Can you work these out from the drawing? Everything is in mm from the part's minimum corner. A direction names the side the tool comes from. Coordinates: 2 decimals unless noted, no trailing zeros. Loops run counter-clockwise (first coordinate to the right, second up) from the corner with the lowest first, then second, coordinate; pieces in that order, holes last. Notation, with made-up numbers: (47.25, 25.25) - (54.25, 25.25) arc R25 ccw to (54.25, 50.25) - close; hole circle Ø6 at (15.5, 54). An arc over 180 degrees is marked (long way). One line per question, with ' | ' between items. Start each with the question number.
1. We'd pull the mould along Z, two halves only. Please class the marked faces 3, 4, 5 and 6: pulls with the +Z half, pulls with the -Z half, needs draft (parallel to the pull), parting line crosses it, or undercut.
2. I want a section at C-C, the plane x = 19.5. Write out the boundary of the cut face in (y, z), then the cut area to 3 significant figures.
3. Please list where these lines run through material, in increasing order: L1, parallel to Z at x = 9, y = 4.75; L2, parallel to X at y = 1.5, z = 10.5; L3, parallel to Z at x = 15, y = 6.75. Write a range as [from, to].
4. I'm going to push flat-ended pins straight in: P1, Ø14, axis at x = 9, z = 10.9, coming from the -Y side; P2, Ø12.5, axis at x = 6.5, z = 14, coming from the -Y side. Where does each tip first touch, or does it pass through?
5. I want a section at D-D, the plane x = 15.9. Write out the boundary of the cut face in (y, z), then the cut area to 3 significant figures.
6. Which directions (+Z, -Z, +X, -X, +Y, -Y) give clear straight access to the entire face, cutting with the end or side of a thin tool? Please do the marked faces 1 and 2.
7. I want a section at A-A, the plane y = 4.5. Write out the boundary of the cut face in (x, z), then the cut area to 3 significant figures.
8. I want a section at B-B, the plane z = 25.9. Write out the boundary of the cut face in (x, y), then the cut area to 3 significant figures.
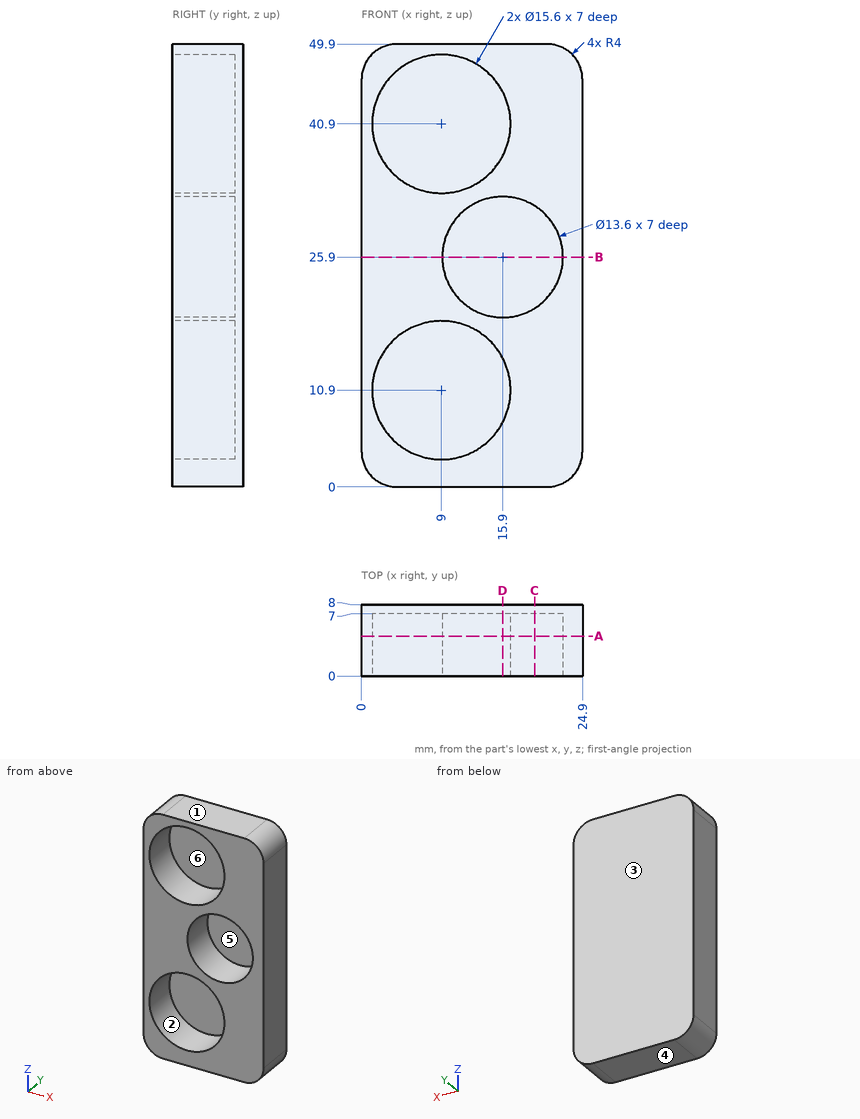
Results are:
1) face 3: needs draft | face 4: pulls with the -Z half | face 5: undercut | face 6: undercut
2) outline: (0, 0) - (8, 0) - (8, 49.9) - (0, 49.9) - (0, 31.67) - (7, 31.67) - (7, 20.13) - (0, 20.13) - close | area: 318 mm2
3) L1: z = [0, 3.1], [18.7, 33.1], [48.7, 49.9] | L2: x = [0, 1.21], [16.79, 24.9] | L3: z = [0, 5.92], [15.88, 19.16], [32.64, 35.92], [45.88, 49.9]
4) P1: stops at y = 7 | P2: stops at y = 0
5) outline: (0, 0) - (8, 0) - (8, 49.9) - (0, 49.9) - (0, 44.54) - (7, 44.54) - (7, 37.26) - (0, 37.26) - (0, 32.7) - (7, 32.7) - (7, 19.1) - (0, 19.1) - (0, 14.54) - (7, 14.54) - (7, 7.26) - (0, 7.26) - close | area: 202 mm2
6) face 1: +Z, +X, -X, +Y, -Y | face 2: -Y
7) outline: (0, 4) arc R4 ccw to (4, 0) - (20.9, 0) arc R4 ccw to (24.9, 4) - (24.9, 45.9) arc R4 ccw to (20.9, 49.9) - (4, 49.9) arc R4 ccw to (0, 45.9) - close; hole circle Ø15.6 at (9, 10.9); hole circle Ø15.6 at (9, 40.9); hole circle Ø13.6 at (15.9, 25.9) | area: 701 mm2
8) outline: (0, 0) - (9.1, 0) - (9.1, 7) - (22.7, 7) - (22.7, 0) - (24.9, 0) - (24.9, 8) - (0, 8) - close | area: 104 mm2
